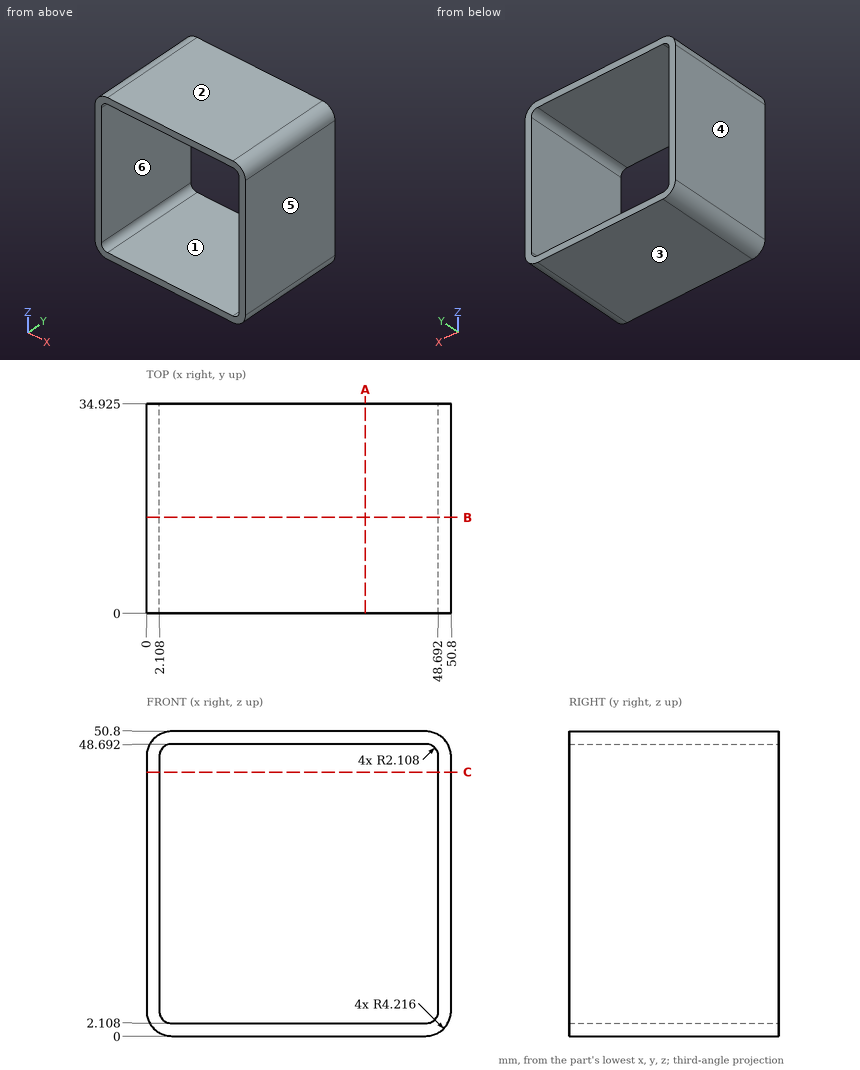
Can you work these out from the drawing? Everything is in mm from the part's minimum corner. A direction names the side the tool comes from. Give positions to 0.01 mm unless a question says otherwise; leave off trailing zeros. Order: outer loops, then holes, each group sorted by start corner. A loop starts at its lowest first (then second) coordinate and runs counter-clockwise, first axis right, second up. Notation, with made-up numbers: M -29,-12 L 17,-12 A28 ccw 17,25 Z; hole C 89.5,20.25 d6. An arc over 180 degrees is marked long. Use a Markdown table: item, result. Add a question column.
Item 1: If I drill on L1, parallel to Z at x = 30, y = 4; L2, parallel to Z at x = 48, y = 6.5 (1 decimal), over which ranges is the centre line in solid material (lowest first)? Write a range as [from, to].
Item 2: For the marked faces 5 and 6, which set-ups out of +Z, -Z, +X, -X, +Y, -Y let a thin tool reach every point of the face, with its end or its side?
Item 3: Will this pin go through, and if not, where does the flat tip stop? pin 1 (17.5 mm diameter, centred on y = 12.5, z = 30.5, fed in from -X).
Item 4: Suppose I cut it at A-A (x = 36.5). List the corners of the cut face in (y, z) for me (1 decimal), then the cut area to 3 significant figures.
Item 5: Suppose I cut it at B-B (y = 16). List the corners of the cut face in (x, z) for me, then the cut area to 3 significant figures.
Item 6: We'd pull the mould along Z, two halves only. Please class the marked faces 1, 2, 3 and 4: +Z half, -Z half, draft (parallel to the pull), parting line (faces both ways), or undercut.
Item 7: Suppose I cut it at C-C (z = 44). List the corners of the cut face in (x, y) for me (1 decimal).
Answer sheet:
| question | item | result |
|---|---|---|
| 1 | L1 | z = [0, 2.11], [48.69, 50.8] |
| 1 | L2 | z = [0.2, 2.7], [48.1, 50.6] |
| 2 | face 5 | +Z, -Z, +X, +Y, -Y |
| 2 | face 6 | +Y, -Y |
| 3 | pin 1 | stops at x = 0 |
| 4 | outline | M 0,0 L 34.9,0 L 34.9,2.1 L 0,2.1 Z; M 0,48.7 L 34.9,48.7 L 34.9,50.8 L 0,50.8 Z |
| 4 | area | 147 mm² |
| 5 | outline | M 0,4.22 A4.22 ccw 4.22,0 L 46.58,0 A4.22 ccw 50.8,4.22 L 50.8,46.58 A4.22 ccw 46.58,50.8 L 4.22,50.8 A4.22 ccw 0,46.58 Z; hole M 2.11,4.22 A2.11 ccw 4.22,2.11 L 46.58,2.11 A2.11 ccw 48.69,4.22 L 48.69,46.58 A2.11 ccw 46.58,48.69 L 4.22,48.69 A2.11 ccw 2.11,46.58 Z |
| 5 | area | 399 mm² |
| 6 | face 1 | undercut |
| 6 | face 2 | +Z half |
| 6 | face 3 | -Z half |
| 6 | face 4 | draft |
| 7 | outline | M 0,0 L 2.1,0 L 2.1,34.9 L 0,34.9 Z; M 48.7,0 L 50.8,0 L 50.8,34.9 L 48.7,34.9 Z |
